Build history of the part. All positions in model axes, mm. Round coordinates to 2 decimals unless told otherwise and drop trailing zeros. Write each loop counter-clockwise with the first axis right and the second up, starting at its lowest first coordinate (ties: lowest second). Pieces come first, ordered by that corner, then holes. Notation, with made-up numbers: (4.25, -6.5) -> (31.25, -6.5) arc R28 ccw to (31.25, 30.5) -> close; hole circle Ø9 at (16, 15). An arc over 180 degrees is marked (long way). One line per question, with ' | ' between items.
from build123d import *

# Parameters (mm, degrees)
SKETCH_1_R          = 3.5
EXTRUDE_1_DEPTH     = 4
FILLET_1_R          = 10
FILLET_2_R          = 2
CUT_EXTRUDE_1_DEPTH = 10
FILLET_3_R          = 1.5
SKETCH_3_R          = 1.5
CUT_EXTRUDE_2_DEPTH = 4


with BuildPart() as part:
    # 草图1 → 凸台-拉伸1 (new body)
    # profile 1 of 2: a face of its own
    with BuildSketch(Plane.XY):
        with BuildLine():
            ThreePointArc((23.201709249, 9.310246395), (0, 25), (-23.201709249, 9.310246395))
            ThreePointArc((-23.201709249, 9.310246395), (-4.741163822, -24.546310631), (25, 0))
            ThreePointArc((25, 0), (24.546310631, 4.741163822), (23.201709249, 9.310246395))
        make_face()
        Circle(SKETCH_1_R, mode=Mode.SUBTRACT)
    # profile 2 of 2: a face of its own
    with BuildSketch(Plane.XY):
        with BuildLine():
            ThreePointArc((25, 0), (-4.741163822, -24.546310631), (-23.201709249, 9.310246395))
            Line((-23.201709249, 9.310246395), (-42.988636962, -40))
            Line((-42.988636962, -40), (-60, -40))
            Line((-60, -40), (-60, -65))
            Line((-60, -65), (60, -65))
            Line((60, -65), (60, -40))
            Line((60, -40), (42.988636962, -40))
            Line((42.988636962, -40), (23.201709249, 9.310246395))
            ThreePointArc((23.201709249, 9.310246395), (24.546310631, 4.741163822), (25, 0))
        make_face()
    extrude(amount=EXTRUDE_1_DEPTH)

    # 圆角1
    fillet_1_edges = [part.edges().sort_by_distance(p)[0] for p in [
        (42.988636962, -40, 2),
        (-42.988636962, -40, 2),
    ]]
    fillet(fillet_1_edges, radius=FILLET_1_R)

    # 圆角2
    fillet_2_edges = [part.edges().sort_by_distance(p)[0] for p in [
        (60, -40, 2),
        (60, -65, 2),
        (-60, -65, 2),
        (-60, -40, 2),
    ]]
    fillet(fillet_2_edges, radius=FILLET_2_R)

    # 草图2 → 切除-拉伸1 (cut)
    with BuildSketch(Plane.XY.offset(4)):
        with BuildLine():
            Line((-43, -61), (-40, -61))
            ThreePointArc((-40, -61), (-41.5, -59.5), (-43, -61))
        make_face()
        with BuildLine():
            ThreePointArc((-60, -63), (-59.414213562, -64.414213562), (-58, -65))
            Line((-58, -65), (-40, -65))
            Line((-40, -65), (-40, -61))
            Line((-40, -61), (-43, -61))
            Line((-43, -61), (-60, -61))
            Line((-60, -61), (-60, -63))
        make_face()
        with BuildLine():
            ThreePointArc((-17, -61), (-18.5, -59.5), (-20, -61))
            Line((-20, -61), (-17, -61))
        make_face()
        Polygon((-20, -61), (-20, -65), (0, -65), (0, -61), (-3, -61), (-17, -61), align=None)
        with BuildLine():
            Line((-3, -61), (0, -61))
            ThreePointArc((0, -61), (-1.5, -59.5), (-3, -61))
        make_face()
        with BuildLine():
            ThreePointArc((23, -61), (21.5, -59.5), (20, -61))
            Line((20, -61), (23, -61))
        make_face()
        Polygon((20, -61), (20, -65), (40, -65), (40, -61), (37, -61), (23, -61), align=None)
        with BuildLine():
            Line((37, -61), (40, -61))
            ThreePointArc((40, -61), (38.5, -59.5), (37, -61))
        make_face()
    extrude(amount=-CUT_EXTRUDE_1_DEPTH, mode=Mode.SUBTRACT)

    # 圆角3
    fillet_3_edges = [part.edges().sort_by_distance(p)[0] for p in [
        (-60, -61, 2),
    ]]
    fillet(fillet_3_edges, radius=FILLET_3_R)

    # 草图3 → 切除-拉伸2 (cut)
    with BuildSketch(Plane.XY.offset(4)):
        with Locations((-55, -58)):
            Circle(SKETCH_3_R)
        with Locations((-35, -58)):
            Circle(SKETCH_3_R)
        with Locations((-15, -58)):
            Circle(SKETCH_3_R)
        with Locations((5, -58)):
            Circle(SKETCH_3_R)
        with Locations((25, -58)):
            Circle(SKETCH_3_R)
        with Locations((45, -58)):
            Circle(SKETCH_3_R)
    extrude(amount=-CUT_EXTRUDE_2_DEPTH, mode=Mode.SUBTRACT)


solid = part.part
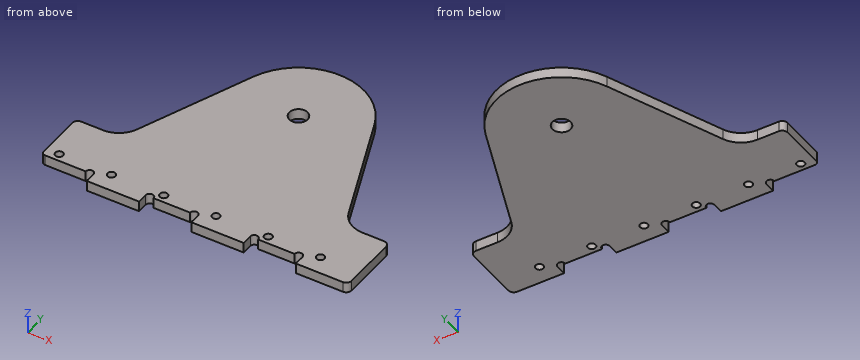
(1) Drop a flat-ended pin along its axis: pin 1 (1.5 mm diameter, centred on y = -27.5, z = 2, fed in from +X). Give the stop position or say it passes through.
Calculated:
pin 1: x = 38.27
(2) Slice it at B-B (y = -58). Write the cut outline in (x, z).
Calculated:
outline: (-60, 0) -> (-56.5, 0) -> (-56.5, 4) -> (-60, 4) -> close; (-53.5, 0) -> (-36.5, 0) -> (-36.5, 4) -> (-53.5, 4) -> close; (-33.5, 0) -> (-16.5, 0) -> (-16.5, 4) -> (-33.5, 4) -> close; (-13.5, 0) -> (3.5, 0) -> (3.5, 4) -> (-13.5, 4) -> close; (6.5, 0) -> (23.5, 0) -> (23.5, 4) -> (6.5, 4) -> close; (26.5, 0) -> (43.5, 0) -> (43.5, 4) -> (26.5, 4) -> close; (46.5, 0) -> (60, 0) -> (60, 4) -> (46.5, 4) -> close
(3) Slice it at A-A (x = -55). Write the cut outline in (y, z).
Calculated:
outline: (-61, 0) -> (-59.5, 0) -> (-59.5, 4) -> (-61, 4) -> close; (-56.5, 0) -> (-40, 0) -> (-40, 4) -> (-56.5, 4) -> close
(4) Wall check: line 1 (Y direction, x = -55, z = 3.25); line 2 (X direction, y = 2, z = 2.1); line 3 (Y direction, x = -51, z = 1.65). Give the ranges that are in metal, low to high. Write a range as from..to.
Calculated:
line 1: -61..-59.5, -56.5..-40 | line 2: -26.14..-2.87, 2.87..26.14 | line 3: -61..-40
(5) Slice it at C-C (z = 1.45). State how many separate pieces and enclosed holes the cut face has, then the cut area to 3 significant figures.
Calculated:
separate pieces: 1 | enclosed holes: 7 | area: 6,470 mm2
(6) Slice it at D-D (x = 45). Write the cut outline in (y, z).
Calculated:
outline: (-65, 0) -> (-59.5, 0) -> (-59.5, 4) -> (-65, 4) -> close; (-56.5, 0) -> (-38.8, 0) -> (-38.8, 4) -> (-56.5, 4) -> close
